Verification items for the finished model (mm, model axes). A direction names the side the tool comes from. Round coordinates to 2 decimals unless told otherwise and drop trailing zeros. Write each loop counter-clockwise with the first axis right and the second up, starting at its lowest first coordinate (ties: lowest second). Pieces come first, ordered by that corner, then holes.
from build123d import *

# Parameters (mm, degrees)
BOSS_EXTRUDE1_DEPTH          = 8.5
SKETCH2_OUTSIDE_W            = 26.636
SKETCH2_OUTSIDE_H            = 26.636
SKETCH2_OUTSIDE_R            = 8
CUT_EXTRUDE1_DEPTH           = 1
CHAMFER2_SIZE                = 0.7
M12_TAPPED_HOLE1_D           = 10.2
M12_TAPPED_HOLE1_DEPTH       = 10
M12_TAPPED_HOLE1_CSINK_D     = 12.05
M12_TAPPED_HOLE1_CSINK_ANGLE = 90
M12_TAPPED_HOLE1_TIP         = 3.064389157
CHAMFER3_SIZE                = 0.7
M3_TAPPED_HOLE5_D            = 2.5
M3_TAPPED_HOLE5_DEPTH        = 7.5
M3_TAPPED_HOLE5_CSINK_D      = 3.05
M3_TAPPED_HOLE5_CSINK_ANGLE  = 90
M3_TAPPED_HOLE5_TIP          = 0.751075774


with BuildPart() as part:
    # Sketch1 → Boss-Extrude1 (new body)
    with BuildSketch(Plane.XY):
        with BuildLine():
            Line((-9.5, 5.545268253), (-9.5, -5.545268253))
            ThreePointArc((-9.5, -5.545268253), (-7.778174593, -7.778174593), (-5.545268253, -9.5))
            Line((-5.545268253, -9.5), (5.545268253, -9.5))
            ThreePointArc((5.545268253, -9.5), (7.778174593, -7.778174593), (9.5, -5.545268253))
            Line((9.5, -5.545268253), (9.5, 5.545268253))
            ThreePointArc((9.5, 5.545268253), (7.778174593, 7.778174593), (5.545268253, 9.5))
            Line((5.545268253, 9.5), (-5.545268253, 9.5))
            ThreePointArc((-5.545268253, 9.5), (-7.778174593, 7.778174593), (-9.5, 5.545268253))
        make_face()
    extrude(amount=-BOSS_EXTRUDE1_DEPTH)

    # Sketch2 outside → Cut-Extrude1 (cut)
    with BuildSketch(Plane.XY):
        Rectangle(SKETCH2_OUTSIDE_W, SKETCH2_OUTSIDE_H)
        Circle(SKETCH2_OUTSIDE_R, mode=Mode.SUBTRACT)
    extrude(amount=-CUT_EXTRUDE1_DEPTH, mode=Mode.SUBTRACT)

    # Chamfer2
    chamfer2_edges = [part.edges().sort_by_distance(p)[0] for p in [
        (-7.778174593, 7.778174593, -8.5),
        (-9.5, 0, -8.5),
        (-7.778174593, -7.778174593, -8.5),
        (0, -9.5, -8.5),
        (7.778174593, -7.778174593, -8.5),
        (9.5, 0, -8.5),
        (0, 9.5, -1),
        (7.778174593, 7.778174593, -1),
        (9.5, 0, -1),
        (7.778174593, -7.778174593, -1),
        (0, -9.5, -1),
        (-7.778174593, -7.778174593, -1),
        (-9.5, 0, -1),
        (-7.778174593, 7.778174593, -1),
        (7.778174593, 7.778174593, -8.5),
        (0, 9.5, -8.5),
    ]]
    chamfer(chamfer2_edges, length=CHAMFER2_SIZE)

    # M12 Tapped Hole1
    with Locations(Plane(origin=(0, 0, -8.5), x_dir=(-1, 0, 0), z_dir=(0, 0, -1))):
        with Locations((0, 0)):
            CounterSinkHole(M12_TAPPED_HOLE1_D / 2, M12_TAPPED_HOLE1_CSINK_D / 2, depth=M12_TAPPED_HOLE1_DEPTH, counter_sink_angle=M12_TAPPED_HOLE1_CSINK_ANGLE)
            with Locations((0, 0, -(M12_TAPPED_HOLE1_DEPTH + M12_TAPPED_HOLE1_TIP / 2))):  # 118° drill point
                Cone(0, M12_TAPPED_HOLE1_D / 2, M12_TAPPED_HOLE1_TIP, mode=Mode.SUBTRACT)

    # Chamfer3
    chamfer3_edges = [part.edges().sort_by_distance(p)[0] for p in [
        (-5.1, 0, 0),
    ]]
    chamfer(chamfer3_edges, length=CHAMFER3_SIZE)

    # M3 Tapped Hole5
    with Locations(Plane(origin=(7.778174593, 7.778174593, -4.5), x_dir=(-0.707106781187, 0.707106781187, 0), z_dir=(0.707106781187, 0.707106781187, 0))):
        with Locations((0, 0)):
            CounterSinkHole(M3_TAPPED_HOLE5_D / 2, M3_TAPPED_HOLE5_CSINK_D / 2, depth=M3_TAPPED_HOLE5_DEPTH, counter_sink_angle=M3_TAPPED_HOLE5_CSINK_ANGLE)
            with Locations((0, 0, -(M3_TAPPED_HOLE5_DEPTH + M3_TAPPED_HOLE5_TIP / 2))):  # 118° drill point
                Cone(0, M3_TAPPED_HOLE5_D / 2, M3_TAPPED_HOLE5_TIP, mode=Mode.SUBTRACT)


solid = part.part
Q1. Material ranges on line 1 along Y through (x, z) = (0, -4); line 2 along Y through (x, z) = (1.5, -2.5), recorded low to high.
Recorded:
line 1: y = -9.5 to -5.1, 5.1 to 9.5
line 2: y = -9.5 to -4.87, 4.87 to 9.5
Q2. Tool access check on faces 5 (the flat face through (-5, 7, -1)), 6 (the conical face through (-7.51, -7.45, -1.28)). Record the directions out of +Z, -Z, +X, -X, +Y, -Y that give a thin tool (end or side, any length) a straight path to the whole face; none if there is none.
Recorded:
face 5: +Z
face 6: +Z, -X, -Y
Q3. Release check for a two-part mould opening along Y. For faces 1 (the cylindrical face through (5.32, 5.7, -5.72)), 2 (the cylindrical face through (-1.73, -7.81, -0.49)), 3 (the flat face through (9.5, 0, -5)), 4 (the conical face through (-7.45, 7.51, -8.22)) record: released by +Y, released by -Y, zero draft, split by the parting line, or undercut.
Recorded:
face 1: undercut
face 2: split by the parting line
face 3: zero draft
face 4: released by +Y
Q4. Sectioned sample at A-A (x = 0). Enter the section's corners in (y, z) (3 decimals), plus the area to 3 significant figures.
Recorded:
outline: (-9.5, -7.8) - (-8.8, -8.5) - (-6.025, -8.5) - (-5.1, -7.575) - (-5.1, -0.7) - (-5.8, 0) - (-8, 0) - (-8, -1) - (-8.8, -1) - (-9.5, -1.7) - close; (5.1, -7.575) - (6.025, -8.5) - (8.8, -8.5) - (9.5, -7.8) - (9.5, -1.7) - (8.8, -1) - (8, -1) - (8, 0) - (5.8, 0) - (5.1, -0.7) - close
area: 69.5 mm2
Q5. Depth check by flat-ended pin: P1, Ø1, axis at y = 6.5, z = -5, coming from the -X side; P2, Ø6, axis at x = 0, y = 0, coming from the -Z side. Enter the tip coordinate at first touch or a pass-through.
Recorded:
P1: stops at x = -9.22
P2: passes through
Q6. Sectioned sample at B-B (z = -2.5). Enter the section's corners in (x, y), plus the area to 3 significant figures.
Recorded:
outline: (-9.5, -5.55) arc R11 ccw to (-5.55, -9.5) - (5.55, -9.5) arc R11 ccw to (9.5, -5.55) - (9.5, 5.55) arc R11 ccw to (5.55, 9.5) - (-5.55, 9.5) arc R11 ccw to (-9.5, 5.55) - close; hole circle Ø10.2 at (0, 0)
area: 253 mm2
